Design review of the part built by this model. Coordinates are the model's own, in mm. A direction names the side the tool comes from. Give positions to 0.01 mm unless a question says otherwise; leave off trailing zeros. Loops run counter-clockwise (first coordinate to the right, second up) from the corner with the lowest first, then second, coordinate; pieces in that order, holes last. Notation, with made-up numbers: (64.5, 60.25) -> (122.5, 60.25) arc R34 ccw to (122.5, 91.25) -> close; hole circle Ø8 at (57.5, 64). An arc over 180 degrees is marked (long way). Use a Markdown table: item, result. Add a question column.
1. For pin 1 Ø6 at (x, y) = (-11.5, -4.5) entering from +Z; pin 2 Ø1.5 at (x, y) = (9.5, -9) entering from -Z; pin 3 Ø3 at (x, y) = (7.5, -16.5) entering from -Z, all flat-tipped, find the tip position at first contact; note any pin that passes through.
2. Add section A-A (y = -15). State the section outline as (x, z) points.
3. To check wall thickness, follow line 1 (X direction, y = -6.5, z = -0.5); line 2 (Z direction, x = -0.5, y = -14); line 3 (Z direction, x = -15.5, y = -19.5). State the ranges of each line that lie inside material, in increasing order.
4. For faces 1 (the flat face through (0, -14, -1.7)), 2 (the flat face through (0, -23, 0)), list the 3-axis set-ups (+Z, -Z, +X, -X, +Y, -Y) from which the entire face can be reached by the end or side of a thin tool; tool diameter is ignored.
5. Add section B-B (y = -3.5). State the section outline as (x, z) points, and give its area (3 significant figures).
6. Add section D-D (z = 12.5). State the section outline as (x, y) points.
7. Draft analysis for pull direction X (two halves, no side actions). For faces 3 (the cylindrical face through (-4.336, -9.86, -19.524)), 4 (the cylindrical face through (-17.894, -21.479, -13.721)), 5 (the flat face through (-20.1, 0, -1.6)), state which applies: pulls with the +X half, pulls with the -X half, needs draft (parallel to the pull), parting line crosses it, or undercut.
8. Add section C-C (x = -10). State the section outline as (y, z) points.
```python
from build123d import *

# Parameters (mm, degrees)
F0_R     = 22.5
F0_R_2   = 20
F1_DEPTH = 20
F2_R     = 22.5489054278
F3_DEPTH = 3
F4_R     = 4.5
F5_DEPTH = 12


with BuildPart() as f1:
    # F0 (on Front) → F1 (new body)
    with BuildSketch(Plane.XZ):
        Circle(F0_R)
        Circle(F0_R_2, mode=Mode.SUBTRACT)
    extrude(amount=F1_DEPTH)

    # F2 (on face) → F3 (join)
    with BuildSketch(Plane.XZ.offset(20)):
        Circle(F2_R)
    extrude(amount=F3_DEPTH)

    # F4 (on face) → F5 (join)
    with BuildSketch(Plane(origin=(0, -20, 0), x_dir=(-1, 0, 0), z_dir=(0, 1, 0))):
        Circle(F4_R)
        with BuildLine():
            ThreePointArc((0, 3), (2.1213203436, 2.1213203436), (3, 0))
            ThreePointArc((3, 0), (2.8649192185, -0.8900774526), (2.4718414189, -1.7))
            ThreePointArc((2.4718414189, -1.7), (0, -3), (-2.4718414189, -1.7))
            ThreePointArc((-2.4718414189, -1.7), (-2.6551836095, 1.3964240044), (0, 3))
        make_face(mode=Mode.SUBTRACT)
        with BuildLine():
            ThreePointArc((-2.4718414189, -1.7), (0, -3), (2.4718414189, -1.7))
            Line((2.4718414189, -1.7), (0, -1.7))
            Line((0, -1.7), (-2.4718414189, -1.7))
        make_face()
    extrude(amount=F5_DEPTH)


solid = f1.part
```
Taken from the geometry:
| question | item | result |
|---|---|---|
| 1 | pin 1 | stops at z = 20.83 |
| 1 | pin 2 | stops at z = -20.73 |
| 1 | pin 3 | stops at z = -21.69 |
| 2 | outline | circle Ø45 at (0, 0); circle Ø9 at (0, 0); hole circle Ø40 at (0, 0); hole (-2.47, -1.7) -> (2.47, -1.7) arc R3 ccw (long way) to start |
| 3 | line 1 | x = -22.49 to -19.99, 19.99 to 22.49 |
| 3 | line 2 | z = -22.49 to -19.99, -4.47 to -1.7, 2.96 to 4.47, 19.99 to 22.49 |
| 3 | line 3 | z = -16.31 to -12.64, 12.64 to 16.31 |
| 4 | face 1 | +Y |
| 4 | face 2 | +Z, -Z, +X, -X, -Y |
| 5 | outline | circle Ø45 at (0, 0); hole circle Ø40 at (0, 0) |
| 5 | area | 334 mm^2 |
| 6 | outline | (-18.77, -23) -> (18.77, -23) -> (18.77, -20) -> (18.71, -20) -> (18.71, 0) -> (15.61, 0) -> (15.61, -20) -> (-15.61, -20) -> (-15.61, 0) -> (-18.71, 0) -> (-18.71, -20) -> (-18.77, -20) -> close |
| 7 | face 3 | undercut |
| 7 | face 4 | parting line crosses it |
| 7 | face 5 | needs draft |
| 8 | outline | (-23, -20.21) -> (-20, -20.21) -> (-20, -20.16) -> (0, -20.16) -> (0, -17.32) -> (-20, -17.32) -> (-20, 17.32) -> (0, 17.32) -> (0, 20.16) -> (-20, 20.16) -> (-20, 20.21) -> (-23, 20.21) -> close |
